from build123d import *

# Parameters (mm, degrees)
SKETCH1_R               = 1
BOSS_EXTRUDE1_DEPTH     = 2
SKETCH3_R               = 3.7
BOSS_EXTRUDE2_DEPTH     = 1.7
BOSS_EXTRUDE3_START     = 1.5
SKETCH4_R               = 3.7
BOSS_EXTRUDE3_DEPTH     = 1.5
SKETCH5_R               = 1.25
CUT_EXTRUDE2_DEPTH      = 34.071626812
SKETCH6_R               = 2.25
CUT_EXTRUDE3_DEPTH      = 2.6
SKETCH7_R               = 2.125
CUT_EXTRUDE4_DEPTH      = 1.3
CORTAR_EXTRUIR1_START   = -2
CROQUIS3_R              = 1
CORTAR_EXTRUIR1_DEPTH   = 2
SALIENTE_EXTRUIR3_DEPTH = 1.5
CORTAR_EXTRUIR2_DEPTH   = 5
CORTAR_EXTRUIR3_DEPTH   = 5
SALIENTE_EXTRUIR4_START = -1.7
SALIENTE_EXTRUIR4_DEPTH = 1.7
CORTAR_EXTRUIR4_DEPTH   = 50
CORTAR_EXTRUIR5_DEPTH   = 50


with BuildPart() as part:
    # Sketch1 → Boss-Extrude1 (new body)
    with BuildSketch(Plane(origin=(0, 0, 0), x_dir=(1, 0, 0), z_dir=(0, 1, 0))):
        with BuildLine():
            Line((0.565718668, 3.631196413), (29.95, 2.5))
            ThreePointArc((29.95, 2.5), (32.45, 0), (29.95, -2.5))
            Line((29.95, -2.5), (0.307337184, -3.662126275))
            ThreePointArc((0.307337184, -3.662126275), (-3.672695956, 0.130113074), (0.565718668, 3.631196413))
        make_face()
        with Locations(Location((29.95, 0, 0), (0, 0, 270))):
            Circle(SKETCH1_R, mode=Mode.SUBTRACT)
    extrude(amount=BOSS_EXTRUDE1_DEPTH)

    # Sketch3 → Boss-Extrude2 (add)
    with BuildSketch(Plane.XZ):
        with Locations(Location((0, 0, 0), (0, 0, 80.620746463))):
            Circle(SKETCH3_R)
    extrude(amount=BOSS_EXTRUDE2_DEPTH)

    # Sketch4 → Boss-Extrude3 (add)
    with BuildSketch(Plane(origin=(0, 2, 0), x_dir=(1, 0, 0), z_dir=(0, 1, 0)).offset(BOSS_EXTRUDE3_START)):
        with Locations(Location((0, 0, 0), (0, 0, 279.379253537))):
            Circle(SKETCH4_R)
    extrude(amount=-BOSS_EXTRUDE3_DEPTH)

    # Sketch5 → Cut-Extrude2 (cut, through all)
    with BuildSketch(Plane(origin=(0, 3.5, 0), x_dir=(1, 0, 0), z_dir=(0, 1, 0))):
        with Locations(Location((0, 0, 0), (0, 0, 270))):
            Circle(SKETCH5_R)
    extrude(amount=-CUT_EXTRUDE2_DEPTH, mode=Mode.SUBTRACT)

    # Sketch6 → Cut-Extrude3 (cut)
    with BuildSketch(Plane.XZ.offset(1.7)):
        with Locations(Location((0, 0, 0), (0, 0, 270))):
            Circle(SKETCH6_R)
    extrude(amount=-CUT_EXTRUDE3_DEPTH, mode=Mode.SUBTRACT)

    # Sketch7 → Cut-Extrude4 (cut)
    with BuildSketch(Plane(origin=(0, 3.5, 0), x_dir=(1, 0, 0), z_dir=(0, 1, 0))):
        with Locations(Location((0, 0, 0), (0, 0, 270))):
            Circle(SKETCH7_R)
    extrude(amount=-CUT_EXTRUDE4_DEPTH, mode=Mode.SUBTRACT)

    # Croquis3 → Cortar-Extruir1 (cut)
    with BuildSketch(Plane(origin=(0, 2, 0), x_dir=(1, 0, 0), z_dir=(0, 1, 0)).offset(CORTAR_EXTRUIR1_START)):
        with Locations(Location((29.95, 0, 0), (0, 0, 270))):
            Circle(CROQUIS3_R)
        with Locations(Location((24.95, 0, 0), (0, 0, 270))):
            Circle(CROQUIS3_R)
        with Locations(Location((19.95, 0, 0), (0, 0, 270))):
            Circle(CROQUIS3_R)
        with Locations(Location((14.95, 0, 0), (0, 0, 270))):
            Circle(CROQUIS3_R)
        with Locations(Location((9.95, 0, 0), (0, 0, 270))):
            Circle(CROQUIS3_R)
    extrude(amount=CORTAR_EXTRUIR1_DEPTH, mode=Mode.SUBTRACT)

    # Croquis5 → Saliente-Extruir3 (add)
    with BuildSketch(Plane(origin=(0, 3.5, 0), x_dir=(1, 0, 0), z_dir=(0, 1, 0))):
        with BuildLine():
            Line((6.7, -0.5), (6.7, 0.5))
            Line((6.7, 0.5), (3.666060556, 0.5))
            ThreePointArc((3.666060556, 0.5), (3.7, 0), (3.666060556, -0.5))
            Line((3.666060556, -0.5), (6.7, -0.5))
        make_face()
        with BuildLine():
            Line((6.112876483, -2.5), (6.112876483, -1.5))
            Line((6.112876483, -1.5), (3.382306905, -1.5))
            ThreePointArc((3.382306905, -1.5), (3.095618131, -2.026610073), (2.727636339, -2.5))
            Line((2.727636339, -2.5), (6.112876483, -2.5))
        make_face()
        with BuildLine():
            Line((6.112876483, 2.5), (6.112876483, 1.5))
            Line((6.112876483, 1.5), (3.382306905, 1.5))
            ThreePointArc((3.382306905, 1.5), (3.095618131, 2.026610073), (2.727636339, 2.5))
            Line((2.727636339, 2.5), (6.112876483, 2.5))
        make_face()
    extrude(amount=-SALIENTE_EXTRUIR3_DEPTH)

    # Croquis7 → Cortar-Extruir2 (cut, symmetric)
    with BuildSketch(Plane.XY.offset(0.5)):
        Polygon((6.7, 2), (4.55777799, 3.5), (6.7, 3.5), align=None)
    extrude(amount=CORTAR_EXTRUIR2_DEPTH, both=True, mode=Mode.SUBTRACT)

    # Croquis8 → Cortar-Extruir3 (cut, symmetric)
    with BuildSketch(Plane.XY.offset(0.5)):
        Polygon((6.112876483, 2.411108312), (6.112876483, 2), (6.7, 2), align=None)
    extrude(amount=CORTAR_EXTRUIR3_DEPTH, both=True, mode=Mode.SUBTRACT)

    # Croquis10 → Saliente-Extruir4 (add)
    with BuildSketch(Plane.XZ.offset(1.7).offset(SALIENTE_EXTRUIR4_START)):
        with BuildLine():
            Line((3.666060556, -0.5), (6.7, -0.5))
            Line((6.7, -0.5), (6.7, 0.5))
            Line((6.7, 0.5), (3.666060556, 0.5))
            ThreePointArc((3.666060556, 0.5), (3.691505388, 0.250575281), (3.7, 0))
            ThreePointArc((3.7, 0), (3.691505388, -0.250575281), (3.666060556, -0.5))
        make_face()
        with BuildLine():
            Line((6.112876483, -1.5), (3.382306905, -1.5))
            ThreePointArc((3.382306905, -1.5), (3.095618131, -2.026610073), (2.727636339, -2.5))
            Line((2.727636339, -2.5), (6.112876483, -2.5))
            Line((6.112876483, -2.5), (6.112876483, -1.5))
        make_face()
        with BuildLine():
            Line((6.112876483, 2.5), (2.727636339, 2.5))
            ThreePointArc((2.727636339, 2.5), (3.095618131, 2.026610073), (3.382306905, 1.5))
            Line((3.382306905, 1.5), (6.112876483, 1.5))
            Line((6.112876483, 1.5), (6.112876483, 2.5))
        make_face()
    extrude(amount=SALIENTE_EXTRUIR4_DEPTH)

    # Croquis11 → Cortar-Extruir4 (cut, symmetric)
    with BuildSketch(Plane.XY.offset(0.5)):
        Polygon((6.7, 0), (4.360150735, -1.7), (6.7, -1.7), align=None)
    extrude(amount=CORTAR_EXTRUIR4_DEPTH, both=True, mode=Mode.SUBTRACT)

    # Croquis12 → Cortar-Extruir5 (cut, symmetric)
    with BuildSketch(Plane.XY.offset(0.5)):
        Polygon((6.112876483, 0), (6.112876483, -0.426570204), (6.7, 0), align=None)
    extrude(amount=CORTAR_EXTRUIR5_DEPTH, both=True, mode=Mode.SUBTRACT)


solid = part.part
Read the model definition and answer for the solid it produces. Units are mm, in the model's axes. A direction names the side the tool comes from. Coordinates: 2 decimals unless noted, no trailing zeros. Order: outer loops, then holes, each group sorted by start corner. A loop starts at its lowest first (then second) coordinate and runs counter-clockwise, first axis right, second up. Notation, with made-up numbers: (57, 75.25) -> (102, 75.25) arc R26 cw to (102, 99.25) -> close; hole circle Ø1 at (70, 21). An arc over 180 degrees is marked (long way). Answer as a JSON object with one key per item and string values.
1) A cutting plane is placed at D-D, the plane x = 19.95. Determine the outline of the cut face in (y, z), plus the area to 3 significant figures.
Model answer:
{"outline": "(0, -2.88) -> (2, -2.88) -> (2, -1) -> (0, -1) -> close; (0, 1) -> (2, 1) -> (2, 2.89) -> (0, 2.89) -> close", "area": "7.55 mm²"}
2) The mould has two halves that part along Y. Classify faces 1 (the face through (5.249, -1.054, 0.007)), 2 (the face through (-3.675, 0.986, -0.043)), 3 (the face through (5, 3, -0.5)): released by +Y, released by -Y, zero draft, split by the parting line, or undercut.
Model answer:
{"face 1": "released by -Y", "face 2": "undercut", "face 3": "zero draft"}
3) Each of these flat-tipped pins is pushed along its axis until it touches: pin 1 (3 mm diameter, centred on x = 19.95, z = 0, fed in from +Y); pin 2 (1.5 mm diameter, centred on x = 15.5, y = 0.5, fed in from +Z); pin 3 (1.9 mm diameter, centred on x = 4, y = -0.5, fed in from +Z). Where does it stop, or does it pass through?
Model answer:
{"pin 1": "stops at y = 2", "pin 2": "stops at z = 3.1", "pin 3": "stops at z = 3.55"}
4) A tool of negligible diameter and unlimited length cuts with its end or side. For faces 4 (the face through (4, 3, -2.5)), 5 (the face through (5, 3, 0.5)), 6 (the face through (4, -1, -2.5)), 7 (the face through (4, 3, 2.5)), 8 (the face through (-1, 0.9, -1)), from which of +Z, -Z, +X, -X, +Y, -Y can it reach the whole face along a straight path? Write none if from no direction.
Model answer:
{"face 4": "-Z, +X, +Y", "face 5": "+X, +Y", "face 6": "-Z, +X, -Y", "face 7": "+Z, +X, +Y", "face 8": "-Y"}
5) A cutting plane is placed at A-A, the plane x = 14.95. Determine the outline of the cut face in (y, z).
Model answer:
{"outline": "(0, -3.08) -> (2, -3.08) -> (2, -1) -> (0, -1) -> close; (0, 1) -> (2, 1) -> (2, 3.09) -> (0, 3.09) -> close"}
6) A cutting plane is placed at C-C, the plane y = 2.95. Determine the outline of the cut face in (x, z) (3 decimals), plus the area to 3 significant figures.
Model answer:
{"outline": "(2.728, -2.5) -> (5.343, -2.5) -> (5.343, -1.5) -> (3.382, -1.5) arc R3.7 ccw to (3.666, -0.5) -> (5.343, -0.5) -> (5.343, 0.5) -> (3.666, 0.5) arc R3.7 ccw to (3.382, 1.5) -> (5.343, 1.5) -> (5.343, 2.5) -> (2.728, 2.5) arc R3.7 ccw (long way) to start; hole circle Ø4.25 at (0, 0)", "area": "35.0 mm²"}
7) A cutting plane is placed at B-B, the plane y = 0.55. Determine the outline of the cut face in (x, z) (3 decimals).
Model answer:
{"outline": "(0.307, 3.662) arc R3.675 ccw (long way) to (0.566, -3.631) -> (29.95, -2.5) arc R2.5 ccw to (29.95, 2.5) -> close; hole circle Ø4.5 at (0, 0); hole circle Ø2 at (9.95, 0); hole circle Ø2 at (14.95, 0); hole circle Ø2 at (19.95, 0); hole circle Ø2 at (24.95, 0); hole circle Ø2 at (29.95, 0)"}
8) Consider line 1 along Y through (x, z) = (9, -1.25); line 2 along X through (y, z) = (3.25, 0) (3 decimals); line 3 along Z through (x, y) = (1, -1.3). Determine where each line is inside the solid, lowest interval first. Write a range as from..to.
Model answer:
{"line 1": "y = 0..2", "line 2": "x = -3.7..-2.125, 2.125..4.915", "line 3": "z = -3.56..-2.02, 2.02..3.56"}
